from build123d import *

# Parameters (mm, degrees)
CROQUIS1_W                   = 90
CROQUIS1_H                   = 90
SALIENTE_EXTRUIR1_DEPTH      = 90
REDONDEO2_R                  = 30
CROQUIS2_R                   = 18
SALIENTE_EXTRUIR2_DEPTH      = 1
SALIENTE_EXTRUIR2_DEPTH_BACK = 12
CORTAR_EXTRUIR1_DEPTH        = 74
CROQUIS4_R                   = 12
SALIENTE_EXTRUIR3_DEPTH      = 1
SALIENTE_EXTRUIR3_DEPTH_BACK = 6
CORTAR_EXTRUIR2_DEPTH        = 100


with BuildPart() as part:
    # Croquis1 → Saliente-Extruir1 (new body)
    with BuildSketch(Plane.XY):
        with Locations((-11.750768053, -2.707538995)):
            Rectangle(CROQUIS1_W, CROQUIS1_H)
    extrude(amount=SALIENTE_EXTRUIR1_DEPTH)

    # Redondeo2
    redondeo2_edges = [part.edges().sort_by_distance(p)[0] for p in [
        (33.249231947, -2.707538995, 90),
        (-11.750768053, 42.292461005, 90),
        (-56.750768053, -2.707538995, 90),
        (-11.750768053, 42.292461005, 0),
        (33.249231947, -2.707538995, 0),
        (-56.750768053, -2.707538995, 0),
        (-11.750768053, -47.707538995, 90),
        (-56.750768053, 42.292461005, 45),
        (33.249231947, 42.292461005, 45),
    ]]
    fillet(redondeo2_edges, radius=REDONDEO2_R)

    # Croquis2 → Saliente-Extruir2 (add, two sides)
    with BuildSketch(Plane.XY.offset(90)) as saliente_extruir2_sk:
        with Locations((8.324186068, -5.35884863)):
            Circle(CROQUIS2_R)
        with Locations((-31.428963697, -5.35884863)):
            Circle(CROQUIS2_R)
    extrude(amount=SALIENTE_EXTRUIR2_DEPTH)
    extrude(saliente_extruir2_sk.sketch, amount=-SALIENTE_EXTRUIR2_DEPTH_BACK)

    # Croquis3 → Cortar-Extruir1 (cut)
    with BuildSketch(Plane(origin=(0, 42.292461005, 0), x_dir=(1, 0, 0), z_dir=(0, 1, 0))):
        with BuildLine():
            ThreePointArc((-50.140421134, -80.34512543), (-39.601859674, -88.210803678), (-26.750768053, -91))
            Line((-26.750768053, -91), (-50.140421134, -91))
            Line((-50.140421134, -91), (-50.140421134, -80.34512543))
        make_face()
        with BuildLine():
            Line((26.638885028, -91), (26.638885028, -80.34512543))
            ThreePointArc((26.638885028, -80.34512543), (16.100323567, -88.210803678), (3.249231947, -91))
            Line((3.249231947, -91), (26.638885028, -91))
        make_face()
    extrude(amount=-CORTAR_EXTRUIR1_DEPTH, mode=Mode.SUBTRACT)

    # Croquis4 → Saliente-Extruir3 (add, two sides)
    with BuildSketch(Plane.XY.offset(91)) as saliente_extruir3_sk:
        with Locations((-31.428963697, -5.35884863)):
            Circle(CROQUIS4_R)
        with Locations((8.324186068, -5.35884863)):
            Circle(CROQUIS4_R)
    extrude(amount=SALIENTE_EXTRUIR3_DEPTH)
    extrude(saliente_extruir3_sk.sketch, amount=-SALIENTE_EXTRUIR3_DEPTH_BACK)

    # Croquis5 → Cortar-Extruir2 (cut)
    with BuildSketch(Plane(origin=(0, 42.292461005, 0), x_dir=(1, 0, 0), z_dir=(0, 1, 0))):
        with BuildLine():
            ThreePointArc((-48.087335127, -83.84849902), (-38.171101485, -89.892741332), (-26.750768053, -92))
            Line((-26.750768053, -92), (-43.428963697, -92))
            Line((-43.428963697, -92), (-48.087335127, -92))
            Line((-48.087335127, -92), (-48.087335127, -83.84849902))
        make_face()
        with BuildLine():
            ThreePointArc((24.585799021, -83.84849902), (14.669565378, -89.892741332), (3.249231947, -92))
            Line((3.249231947, -92), (19.927427591, -92))
            Line((19.927427591, -92), (24.585799021, -92))
            Line((24.585799021, -92), (24.585799021, -83.84849902))
        make_face()
    extrude(amount=-CORTAR_EXTRUIR2_DEPTH, mode=Mode.SUBTRACT)


solid = part.part
The listing builds one solid part. Answer for the finished solid, in the listing's coordinates (mm). A direction names the side the tool comes from. Give positions to 0.01 mm unless a question says otherwise; leave off trailing zeros. Write each loop counter-clockwise with the first axis right and the second up, starting at its lowest first coordinate (ties: lowest second). Pieces come first, ordered by that corner, then holes. Notation, with made-up numbers: (44.5, -13) - (97.5, -13) arc R24 ccw to (97.5, 22) - close; hole circle Ø6 at (89, 62). An arc over 180 degrees is marked (long way). One line per question, with ' | ' between items. Start each with the question number.
1. Section B-B, the plane z = 37 is taken. Determine the outline of the cut face in (x, y).
2. Straight lines are drawn through the part: line 1 (Z direction, x = 19.5, y = 11); line 2 (Z direction, x = 22, y = 8.5); line 3 (Y direction, x = 6.5, z = 36.5). For each, find the intervals that lie inside material, in ascending order.
3. Section C-C, the plane x = -30 is taken. Determine the outline of the cut face in (y, z).
4. For faces 1 (the face through (-45.386, -16.726, 84.452)), 2 (the face through (-11.541, 33.738, 9.021)), determine the directions among +Z, -Z, +X, -X, +Y, -Y from which every point of the face is accessible in a straight line to the end or side of a thin tool.
5. Section A-A, the plane y = -36 is taken. Determine the outline of the cut face in (x, z).
6. Determine the mould class of faces 3 (the face through (-52.67, -17.29, 75.11)), 4 (the face through (24.694, -17.288, 9.021)), 5 (the face through (-19, -5, 91)), 6 (the face through (-24, -5, 92)) for opening direction X: +X half, -X half, draft (parallel to the pull), parting line (faces both ways), or undercut.
7. Section D-D, the plane y = -14 is taken. Determine the outline of the cut face in (x, z), then the cut area to 3 significant figures.
8. Given P1, Ø1.5, axis at y = -37.5, z = 26.5, coming from the -X side; P2, Ø5, axis at y = 17.5, z = 43, coming from the +X side; P3, Ø4, axis at x = -17, y = -7, coming from the +Z side, each flat-ended and moving along its own axis, determine where each tip first touches the part or whether it passes through.
Result:
1) outline: (-56.75, -47.71) - (33.25, -47.71) - (33.25, 12.29) arc R30 ccw to (3.25, 42.29) - (-26.75, 42.29) arc R30 ccw to (-56.75, 12.29) - close
2) line 1: z = 4.78 to 85.22 | line 2: z = 6.58 to 83.42 | line 3: y = -47.71 to 42.12
3) outline: (-47.71, 0.18) - (12.29, 0.18) arc R29.82 ccw to (42.12, 30) - (42.12, 60) arc R29.82 ccw to (12.58, 89.82) - (12.58, 90.83) - (6.56, 90.83) - (6.56, 91.83) - (-17.27, 91.83) - (-17.27, 90.83) - (-23.3, 90.83) - (-23.3, 89.47) arc R30 ccw to (-47.71, 60) - close
4) face 1: +Z | face 2: -Z, +X, -X, +Y
5) outline: (-56.75, 30) arc R30 ccw to (-26.75, 0) - (3.25, 0) arc R30 ccw to (33.25, 30) - (33.25, 60) arc R30 ccw to (21.54, 83.78) - (-45.04, 83.78) arc R30 ccw to (-56.75, 60) - close
6) face 3: -X half | face 4: +X half | face 5: undercut | face 6: draft
7) outline: (-56.75, 30) arc R30 ccw to (-26.75, 0) - (3.25, 0) arc R30 ccw to (33.25, 30) - (33.25, 60) arc R30 ccw to (24.11, 81.56) - (24.11, 82.93) arc R31 ccw to (16.65, 87.95) - (16.65, 89.06) arc R32 ccw to (3.25, 92) - (0, 92) - (0, 91) - (-7.47, 91) - (-7.47, 90) - (-15.64, 90) - (-15.64, 91) - (-23.1, 91) - (-23.1, 92) - (-26.75, 92) arc R32 ccw to (-39.76, 89.24) - (-39.76, 88.14) arc R31 ccw to (-47.22, 83.28) - (-47.22, 81.93) arc R30 ccw to (-56.75, 60) - close | area: 7,430 mm2
8) P1: stops at x = -56.62 | P2: stops at x = 33.13 | P3: stops at z = 91
